Geometry: final body of the model. Coordinates: model frame, mm. A direction names the side the tool comes from. Give positions to 0.01 mm unless a question says otherwise; leave off trailing zeros. Loops run counter-clockwise (first coordinate to the right, second up) from the corner with the lowest first, then second, coordinate; pieces in that order, holes last. Notation, with made-up numbers: (55, 19.25) - (60, 19.25) arc R12 cw to (60, 26.25) - close; hole circle Ø8 at (-21.75, -2). An arc over 180 degrees is marked (long way). Use one line per item in the form item = value.
```python
from build123d import *

# Parameters (mm, degrees)
SKETCH_2_W          = 10
SKETCH_2_H          = 130
EXTRUDE_1_DEPTH     = 15
SKETCH_3_R          = 1.5
CUT_EXTRUDE_1_DEPTH = 220.82947937
SKETCH_4_R          = 2.5
CUT_EXTRUDE_2_DEPTH = 7
SKETCH_5_R          = 2.5
CUT_EXTRUDE_3_DEPTH = 179.168652345


with BuildPart() as part:
    # 草图2 → 凸台-拉伸1 (new body)
    with BuildSketch(Plane(origin=(0, 0, 0), x_dir=(1, 0, 0), z_dir=(0, 1, 0))):
        Polygon((0, 73.064516129), (-85, 73.064516129), (-85, 63.064516129), (-75, 63.064516129), (0, 63.064516129), align=None)
        Polygon((-160, 73.064516129), (-160, 63.064516129), (-150, 63.064516129), (-85, 63.064516129), (-85, 73.064516129), align=None)
        with Locations((-80, -1.935483871)):
            Rectangle(SKETCH_2_W, SKETCH_2_H)
        Polygon((-85, -66.935483871), (-85, -76.935483871), (0, -76.935483871), (0, -66.935483871), (-75, -66.935483871), align=None)
        Polygon((-150, -66.935483871), (-160, -66.935483871), (-160, -76.935483871), (-85, -76.935483871), (-85, -66.935483871), align=None)
        with Locations((-155, -1.935483871)):
            Rectangle(SKETCH_2_W, SKETCH_2_H)
    extrude(amount=EXTRUDE_1_DEPTH)

    # 草图3 → 切除-拉伸1 (cut, through all)
    with BuildSketch(Plane.XY.offset(76.935483871)):
        with Locations((-5, 12)):
            Circle(SKETCH_3_R)
        with Locations((-5, 3)):
            Circle(SKETCH_3_R)
        with Locations((-15, 12)):
            Circle(SKETCH_3_R)
        with Locations((-15, 3)):
            Circle(SKETCH_3_R)
    extrude(amount=-CUT_EXTRUDE_1_DEPTH, mode=Mode.SUBTRACT)

    # 草图4 → 切除-拉伸2 (cut)
    with BuildSketch(Plane.ZY.offset(160)):
        with Locations((-63.064516129, 7.5)):
            Circle(SKETCH_4_R)
        with Locations((-13.064516129, 7.5)):
            Circle(SKETCH_4_R)
        with Locations((16.935483871, 7.5)):
            Circle(SKETCH_4_R)
        with Locations((66.935483871, 7.5)):
            Circle(SKETCH_4_R)
    extrude(amount=-CUT_EXTRUDE_2_DEPTH, mode=Mode.SUBTRACT)

    # 草图5 → 切除-拉伸3 (cut, through all)
    with BuildSketch(Plane(origin=(0, 15, 0), x_dir=(1, 0, 0), z_dir=(0, 1, 0))):
        with Locations(Location((-10, 68.064516129, 0), (0, 0, 270))):
            Circle(SKETCH_5_R)
        with Locations(Location((-10, -71.935483871, 0), (0, 0, 270))):
            Circle(SKETCH_5_R)
    extrude(amount=-CUT_EXTRUDE_3_DEPTH, mode=Mode.SUBTRACT)


solid = part.part
```
(1) Access query for faces 4 (the face through (-150, 7, 3)), 5 (the face through (-153, 8, 17)), 6 (the face through (-38, 7, -63.065)). Directions: +Z, -Z, +X, -X, +Y, -Y. A direction counts if a zero-diameter tool reaches every point of the face in a straight line with its end or side. Return the directions, or none.
Solution:
face_4 = +Y, -Y
face_5 = -X
face_6 = +X, +Y, -Y
(2) Cut plane A-A (x = -119). Return the cut outline in (y, z).
Solution:
outline = (0, -73.06) - (15, -73.06) - (15, -63.06) - (0, -63.06) - close; (0, 66.94) - (15, 66.94) - (15, 76.94) - (0, 76.94) - close
(3) Pin query (flat end, axial travel): P1, Ø2.5, axis at x = -15, y = 3, coming from the +Z side; P2, Ø6, axis at y = 13, z = 47.5, coming from the +X side; P3, Ø4, axis at y = 7.5, z = -63.06, coming from the -X side. Return the tip coordinate at first contact, or that it passes through.
Solution:
P1 = through
P2 = -75
P3 = -153
(4) Material intervals for L1, parallel to Y at x = -15, z = 71; L2, parallel to Z at x = -116.5, y = 2.75; L3, parallel to X at y = 6.5, z = 66, sorted ascending. Write a range as from..to.
Solution:
L1 = 0..1.5, 4.5..10.5, 13.5..15
L2 = -73.06..-63.06, 66.94..76.94
L3 = -153..-150, -85..-75
(5) Cut plane B-B (z = -36). Return the cut outline in (x, y).
Solution:
outline = (-160, 0) - (-150, 0) - (-150, 15) - (-160, 15) - close; (-85, 0) - (-75, 0) - (-75, 15) - (-85, 15) - close
(6) Cut plane C-C (x = -10). Return the cut outline in (y, z).
Solution:
outline = (0, -73.06) - (15, -73.06) - (15, -70.56) - (0, -70.56) - close; (0, -65.56) - (15, -65.56) - (15, -63.06) - (0, -63.06) - close; (0, 66.94) - (15, 66.94) - (15, 69.44) - (0, 69.44) - close; (0, 74.44) - (15, 74.44) - (15, 76.94) - (0, 76.94) - close
(7) Pull-direction query (Z, two-part tool) for faces 1 (the face through (-11.52, 7.6, 69.95)), 2 (the face through (-81, 15, 1)), 3 (the face through (-79, 7, -73.065)); classes: released by +Z, released by -Z, zero draft, split by the parting line, or undercut.
Solution:
face_1 = undercut
face_2 = zero draft
face_3 = released by -Z
(8) Cut plane D-D (y = 7.5). Give the number of separate pieces and of enclosed holes in the cut face, plus the area to 3 significant figures.
Solution:
separate_pieces = 1
enclosed_holes = 3
area = 5,620 mm2
